from build123d import *

# Parameters (mm, degrees)
SKETCH1_W           = 50.8
SKETCH1_H           = 50.8
BOSS_EXTRUDE1_DEPTH = 4.7625
SKETCH2_W           = 50.8
SKETCH2_H           = 50.8
SKETCH2_W_2         = 25.4
SKETCH2_H_2         = 25.4
SKETCH2_R           = 1.00076
SKETCH2_R_2         = 1.09982
SKETCH2_R_3         = 1.15062
SKETCH2_R_4         = 1.24968
CUT_EXTRUDE1_DEPTH  = 5.7625
CUT_EXTRUDE2_DEPTH  = 5.7625


with BuildPart() as part:
    # Sketch1 → Boss-Extrude1 (new body)
    with BuildSketch(Plane(origin=(0, 0, 0), x_dir=(1, 0, 0), z_dir=(0, 1, 0))):
        Rectangle(SKETCH1_W, SKETCH1_H)
    extrude(amount=BOSS_EXTRUDE1_DEPTH)

    # Sketch2 → Cut-Extrude1 (cut, through all)
    with BuildSketch(Plane(origin=(0, 4.7625, 0), x_dir=(1, 0, 0), z_dir=(0, 1, 0))):
        Rectangle(SKETCH2_W, SKETCH2_H)
        Rectangle(SKETCH2_W_2, SKETCH2_H_2, mode=Mode.SUBTRACT)
        with Locations((-6.35, 6.35)):
            Circle(SKETCH2_R)
        with Locations((6.35, 6.35)):
            Circle(SKETCH2_R_2)
        with Locations((-6.35, -6.35)):
            Circle(SKETCH2_R_3)
        with Locations((6.35, -6.35)):
            Circle(SKETCH2_R_4)
    extrude(amount=-CUT_EXTRUDE1_DEPTH, mode=Mode.SUBTRACT)

    # Sketch3 → Cut-Extrude2 (cut, through all)
    with BuildSketch(Plane(origin=(0, 4.7625, 0), x_dir=(1, 0, 0), z_dir=(0, 1, 0))):
        Polygon((-10.414075549, 12.7), (-12.7, 12.7), (-12.7, 10.750584792), align=None)
    extrude(amount=-CUT_EXTRUDE2_DEPTH, mode=Mode.SUBTRACT)


solid = part.part
Source: CAD feature listing. Evaluate the final solid. Frame: model axes, mm. Round coordinates to 2 decimals unless told otherwise and drop trailing zeros. Loops run counter-clockwise (first coordinate to the right, second up) from the corner with the lowest first, then second, coordinate; pieces in that order, holes last.
Q1. Mould query, pull axis Z, two halves, no side actions, for faces 1 (the face through (-11.573, 2.415, -11.712)), 2 (the face through (-7.088, 2.415, -7.026)), 3 (the face through (12.7, 2, 0)), 4 (the face through (7.366, 2.415, -5.929)). Classes: pulls with the +Z half, pulls with the -Z half, needs draft (parallel to the pull), parting line crosses it, or undercut.
Q2. Ray query, line 1 (X direction, y = 3.4, z = 6.35); line 2 (Z direction, x = 6.35, y = 2); line 3 (Z direction, x = -6.35, y = 2.85). Return the intervals inside material, ascending.
Q3. Section C-C, the plane y = 1.6. Return loops of the section in (x, z).
Q4. Section A-A, the plane x = -6.35. Return loops of the section in (y, z).
Q5. Section B-B, the plane z = -6.35. Return loops of the section in (x, y).
Solutions:
1. face 1: pulls with the -Z half
1. face 2: undercut
1. face 3: needs draft
1. face 4: undercut
2. line 1: x = -12.7 to -7.5, -5.2 to 5.1, 7.6 to 12.7
2. line 2: z = -12.7 to -7.45, -5.25 to 5.1, 7.6 to 12.7
2. line 3: z = -12.7 to -7.35, -5.35 to 5.2, 7.5 to 12.7
3. outline: (-12.7, -10.75) - (-10.41, -12.7) - (12.7, -12.7) - (12.7, 12.7) - (-12.7, 12.7) - close; hole circle Ø2.3 at (-6.35, 6.35); hole circle Ø2 at (-6.35, -6.35); hole circle Ø2.5 at (6.35, 6.35); hole circle Ø2.2 at (6.35, -6.35)
4. outline: (0, -12.7) - (4.76, -12.7) - (4.76, -7.35) - (0, -7.35) - close; (0, -5.35) - (4.76, -5.35) - (4.76, 5.2) - (0, 5.2) - close; (0, 7.5) - (4.76, 7.5) - (4.76, 12.7) - (0, 12.7) - close
5. outline: (-12.7, 0) - (-7.35, 0) - (-7.35, 4.76) - (-12.7, 4.76) - close; (-5.35, 0) - (5.25, 0) - (5.25, 4.76) - (-5.35, 4.76) - close; (7.45, 0) - (12.7, 0) - (12.7, 4.76) - (7.45, 4.76) - close
